from build123d import *

# Parameters (mm, degrees)
BOX001_W          = 10
BOX001_H          = 10
BOX001_DEPTH      = 10
CYLINDER002_R     = 3.5
CYLINDER002_DEPTH = 12


with BuildPart() as obj1:
    # Box001 → Box001 (new body)
    with BuildSketch(Plane(origin=(2, -1.5, 15), x_dir=(1, 0, 0), z_dir=(0, 0, 1))):
        with Locations((5, 5)):
            Rectangle(BOX001_W, BOX001_H)
    extrude(amount=BOX001_DEPTH)


with BuildPart() as cut:
    # Cylinder002 → Cylinder002 (new body)
    with BuildSketch(Plane(origin=(7.5, -2.5, 13), x_dir=(1, 0, 0), z_dir=(0, 0, 1))):
        Circle(CYLINDER002_R)
    extrude(amount=CYLINDER002_DEPTH)

    # Cut: cut obj1
    add(obj1.part, mode=Mode.SUBTRACT)


solid = cut.part
Work out the finished part from the listing and answer in its coordinate system (mm). A direction names the side the tool comes from. Give positions to 0.01 mm unless a question says otherwise; leave off trailing zeros. Loops run counter-clockwise (first coordinate to the right, second up) from the corner with the lowest first, then second, coordinate; pieces in that order, holes last. Notation, with made-up numbers: (36, 22.5) -> (49, 22.5) arc R19 cw to (49, 31.5) -> close; hole circle Ø1 at (60.25, 55). An arc over 180 degrees is marked (long way). Use a Markdown table: item, result. Add a question column.
1. Section A-A on x = 7.5 is taken. Determine the outline of the cut face in (y, z).
2. Section C-C on z = 16 is taken. Determine the outline of the cut face in (x, y), and give its area (3 significant figures).
3. Section D-D on x = 10 is taken. Determine the outline of the cut face in (y, z).
4. Find the intervals of material crossed by probe 1 along Z at (x, y) = (8.25, -0.5); probe 2 along X at (y, z) = (-3.5, 23.5); probe 3 along X at (y, z) = (-4.75, 24), in increasing order.
5. Flat-ended cylindrical pins translate along their axes: pin 1 Ø1 at (x, z) = (8.5, 20) entering from -Y; pin 2 Ø2 at (x, z) = (6.5, 19.5) entering from +Y; pin 3 Ø1 at (y, z) = (-3.5, 17) entering from +X. Find the tip coordinate at first contact, or state that the pin passes through.
6. Section B-B on y = -3.5 is taken. Determine the outline of the cut face in (x, z), and give its area (3 significant figures).
7. For faces 1 (the flat face through (7, -3, 25)), 2 (the flat face through (7, -1, 15)), determine the directions among +Z, -Z, +X, -X, +Y, -Y from which every point of the face is accessible in a straight line to the end or side of a thin tool.
Results below:
| question | item | result |
|---|---|---|
| 1 | outline | (-6, 13) -> (1, 13) -> (1, 15) -> (-1.5, 15) -> (-1.5, 25) -> (-6, 25) -> close |
| 2 | outline | (4.15, -1.5) arc R3.5 ccw (long way) to (10.85, -1.5) -> close |
| 2 | area | 26.1 mm^2 |
| 3 | outline | (-4.95, 13) -> (-0.05, 13) -> (-0.05, 15) -> (-1.5, 15) -> (-1.5, 25) -> (-4.95, 25) -> close |
| 4 | probe 1 | z = 13 to 15 |
| 4 | probe 2 | x = 4.15 to 10.85 |
| 4 | probe 3 | x = 4.82 to 10.18 |
| 5 | pin 1 | stops at y = -5.96 |
| 5 | pin 2 | stops at y = -1.5 |
| 5 | pin 3 | stops at x = 10.96 |
| 6 | outline | (4.15, 13) -> (10.85, 13) -> (10.85, 25) -> (4.15, 25) -> close |
| 6 | area | 80.5 mm^2 |
| 7 | face 1 | +Z, +X, -X, +Y, -Y |
| 7 | face 2 | +Z, +X, -X, +Y |
